from build123d import *

# Parameters (mm, degrees)
F0_W     = 90
F0_H     = 120
F1_DEPTH = 30
F2_T     = -2.5
F3_R     = 1.55
F4_DEPTH = 25


with BuildPart() as f1:
    # F0 (on Front) → F1 (new body)
    with BuildSketch(Plane.XZ):
        Rectangle(F0_W, F0_H)
    extrude(amount=F1_DEPTH)

    # F2
    f2_openings = [f1.faces().sort_by_distance(p)[0] for p in [
        (0, -30, 0),
    ]]
    offset(amount=F2_T, openings=f2_openings)

    # F3 (on face) → F4 (cut)
    with BuildSketch(Plane(origin=(0, 0, -60), x_dir=(1, 0, 0), z_dir=(0, 0, -1))):
        with Locations((0, 15)):
            Circle(F3_R)
    extrude(amount=-F4_DEPTH, mode=Mode.SUBTRACT)


solid = f1.part
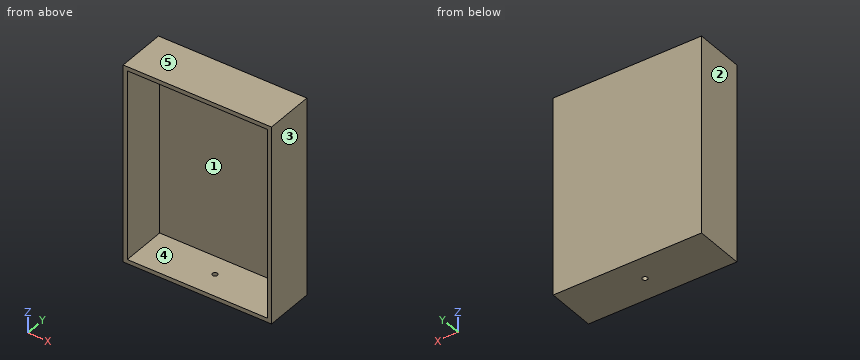
Here's how the part is built. I have some questions about the finished solid (model axes, mm). Face numbers are marked on the shaded views. A direction names the side the tool comes from. Give positions to 0.01 mm unless a question says otherwise; leave off trailing zeros. Order: outer loops, then holes, each group sorted by start corner. A loop starts at its lowest first (then second) coordinate and runs counter-clockwise, first axis right, second up. Notation, with made-up numbers: (-39.5, 56.25) -> (-4.5, 56.25) arc R28 cw to (-4.5, 80.25) -> close; hole circle Ø9 at (-22, 83.25). An arc over 180 degrees is marked (long way). Use a Markdown table: item, result. Add a question column.
Item 1: Imagine slicing it at A-A on x = 0. Please give me the cut outline in (y, z).
Item 2: I need wall thicknesses on line 1 (Z direction, x = 41, y = -20); line 2 (Y direction, x = 0, z = -58); line 3 (X direction, y = -16.5, z = -28). Which ranges of each line are inside material? Lowest first, please.
Item 3: Imagine slicing it at D-D on y = -15. Please give me the cut outline in (x, z).
Item 4: For the marked faces 1 and 2, which set-ups out of +Z, -Z, +X, -X, +Y, -Y let a thin tool reach every point of the face, with its end or its side?
Item 5: If we mould it in two halves opening along Z, with no side actions, what happens to the marked faces 3, 4 and 5? For each: pulls with the +Z half, pulls with the -Z half, needs draft (parallel to the pull), parting line crosses it, or undercut.
Item 6: Will these pins go through, and if not, where does the flat tip stop? pin 1 (8 mm diameter, centred on x = 7, z = -5.5, fed in from +Y); pin 2 (12 mm diameter, centred on x = 26.5, z = 7.5, fed in from -Y).
Item 7: Imagine slicing it at B-B on y = -21.75. Please give me the cut outline in (x, z), plus the area to 4 significant figures.
Item 8: Imagine slicing it at C-C on x = -25.5. Please give me the cut outline in (y, z), plus the area to 4 significant figures.
Data:
| question | item | result |
|---|---|---|
| 1 | outline | (-30, -60) -> (-16.55, -60) -> (-16.55, -57.5) -> (-30, -57.5) -> close; (-30, 57.5) -> (-2.5, 57.5) -> (-2.5, -57.5) -> (-13.45, -57.5) -> (-13.45, -60) -> (0, -60) -> (0, 60) -> (-30, 60) -> close |
| 2 | line 1 | z = -60 to -57.5, 57.5 to 60 |
| 2 | line 2 | y = -30 to -16.55, -13.45 to 0 |
| 2 | line 3 | x = -45 to -42.5, 42.5 to 45 |
| 3 | outline | (-45, -60) -> (-1.55, -60) -> (-1.55, -57.5) -> (-42.5, -57.5) -> (-42.5, 57.5) -> (42.5, 57.5) -> (42.5, -57.5) -> (1.55, -57.5) -> (1.55, -60) -> (45, -60) -> (45, 60) -> (-45, 60) -> close |
| 4 | face 1 | -Y |
| 4 | face 2 | +Z, -Z, -X, +Y, -Y |
| 5 | face 3 | needs draft |
| 5 | face 4 | undercut |
| 5 | face 5 | pulls with the +Z half |
| 6 | pin 1 | stops at y = 0 |
| 6 | pin 2 | stops at y = -2.5 |
| 7 | outline | (-45, -60) -> (45, -60) -> (45, 60) -> (-45, 60) -> close; hole (-42.5, -57.5) -> (42.5, -57.5) -> (42.5, 57.5) -> (-42.5, 57.5) -> close |
| 7 | area | 1,025 mm² |
| 8 | outline | (-30, -60) -> (0, -60) -> (0, 60) -> (-30, 60) -> (-30, 57.5) -> (-2.5, 57.5) -> (-2.5, -57.5) -> (-30, -57.5) -> close |
| 8 | area | 437.5 mm² |
